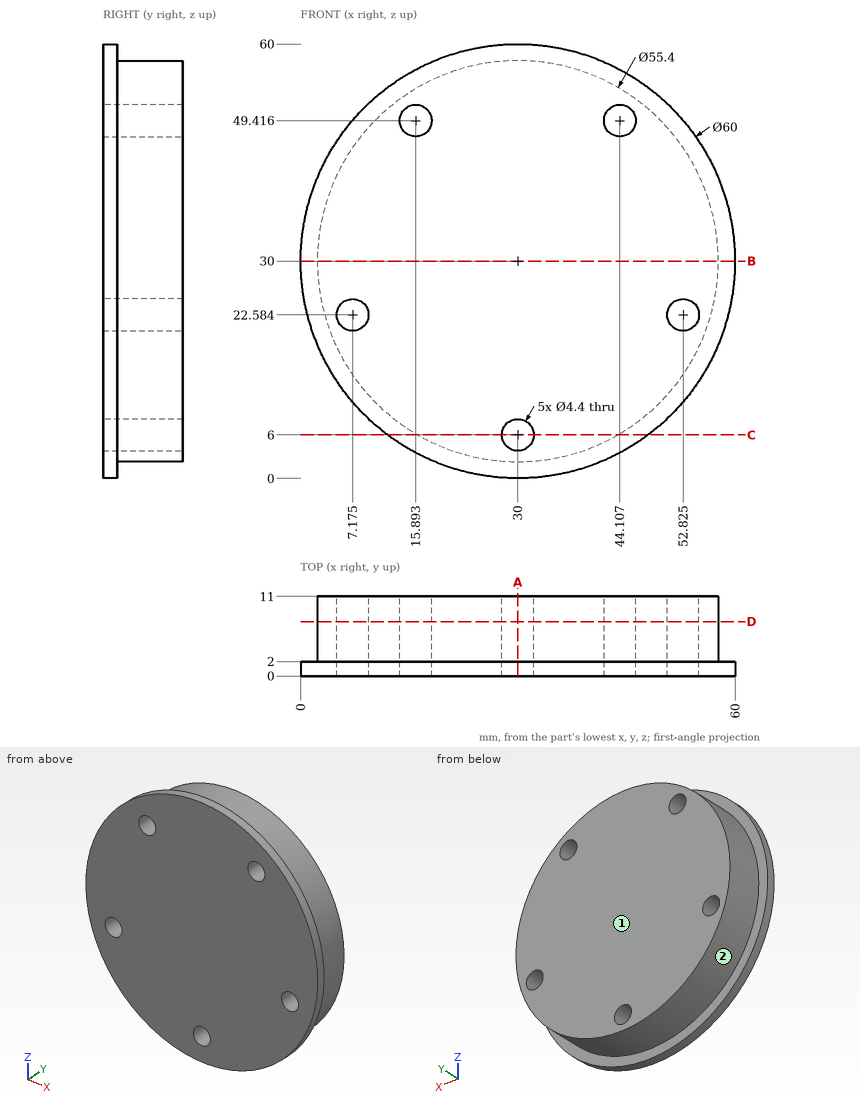
Could you check a few things on this drawing? It's one solid part, dimensions in mm from its lowest x, y, z. A direction names the side the tool comes from. Give positions to 0.01 mm unless a question says otherwise; leave off trailing zeros. Order: outer loops, then holes, each group sorted by start corner. A loop starts at its lowest first (then second) coordinate and runs counter-clockwise, first axis right, second up. Notation, with made-up numbers: (-28.75, 27) - (19.25, 27) arc R16 cw to (19.25, 42) - close; hole circle Ø11 at (-31.75, 12.5). An arc over 180 degrees is marked (long way). One line per item, written item: value. Start each with the question number.
1. For the marked faces 1 and 2, which set-ups out of +Z, -Z, +X, -X, +Y, -Y let a thin tool reach every point of the face, with its end or its side?
2. Imagine slicing it at A-A on x = 30. List the corners of the cut face in (y, z) for me.
3. Imagine slicing it at C-C on z = 6. List the corners of the cut face in (x, y) for me.
4. Imagine slicing it at B-B on z = 30. List the corners of the cut face in (x, y) for me.
5. Imagine slicing it at D-D on y = 7.5. List the corners of the cut face in (x, z) for me (1 decimal).
6. For P1, Ø5, axis at x = 52, y = 1.5, coming from the +Z side; P2, Ø6, axis at x = 25.5, y = 9.5, coming from the +Z side; P3, Ø1, axis at y = 5.5, z = 37, coming from the -X side, each with a flat end and sliding along its axis, tell me the tip position at first contact or that it passes through.
7. If I drill on probe 1 along X at (y, z) = (5.5, 50.5); probe 2 along X at (y, z) = (5, 49) (1 decimal); probe 3 along Z at (x, y) = (28, 2.25) (1 decimal), over which ranges is the centre line in solid material (lowest first)?
Values:
1. face 1: +Z, -Z, +X, -X, +Y
1. face 2: +Y
2. outline: (0, 0) - (2, 0) - (2, 2.3) - (11, 2.3) - (11, 3.8) - (0, 3.8) - close; (0, 8.2) - (11, 8.2) - (11, 57.7) - (2, 57.7) - (2, 60) - (0, 60) - close
3. outline: (12, 0) - (27.8, 0) - (27.8, 11) - (16.17, 11) - (16.17, 2) - (12, 2) - close; (32.2, 0) - (48, 0) - (48, 2) - (43.83, 2) - (43.83, 11) - (32.2, 11) - close
4. outline: (0, 0) - (60, 0) - (60, 2) - (57.7, 2) - (57.7, 11) - (2.3, 11) - (2.3, 2) - (0, 2) - close
5. outline: circle Ø55.4 at (30, 30); hole circle Ø4.4 at (7.2, 22.6); hole circle Ø4.4 at (15.9, 49.4); hole circle Ø4.4 at (30, 6); hole circle Ø4.4 at (44.1, 49.4); hole circle Ø4.4 at (52.8, 22.6)
6. P1: z = 52.8
6. P2: z = 57.66
6. P3: x = 3.07
7. probe 1: 11.37 to 13.98, 17.81 to 42.19, 46.02 to 48.63
7. probe 2: 9.8 to 13.7, 18.1 to 41.9, 46.3 to 50.2
7. probe 3: 2.4 to 5.1, 6.9 to 57.6
